The figure shows three views and two pictorial views of one solid part (mm, origin at its lowest corner). Answer the questions. Coordinates: 2 decimals unless noted, no trailing zeros. Loops run counter-clockwise (first coordinate to the right, second up) from the corner with the lowest first, then second, coordinate; pieces in that order, holes last.
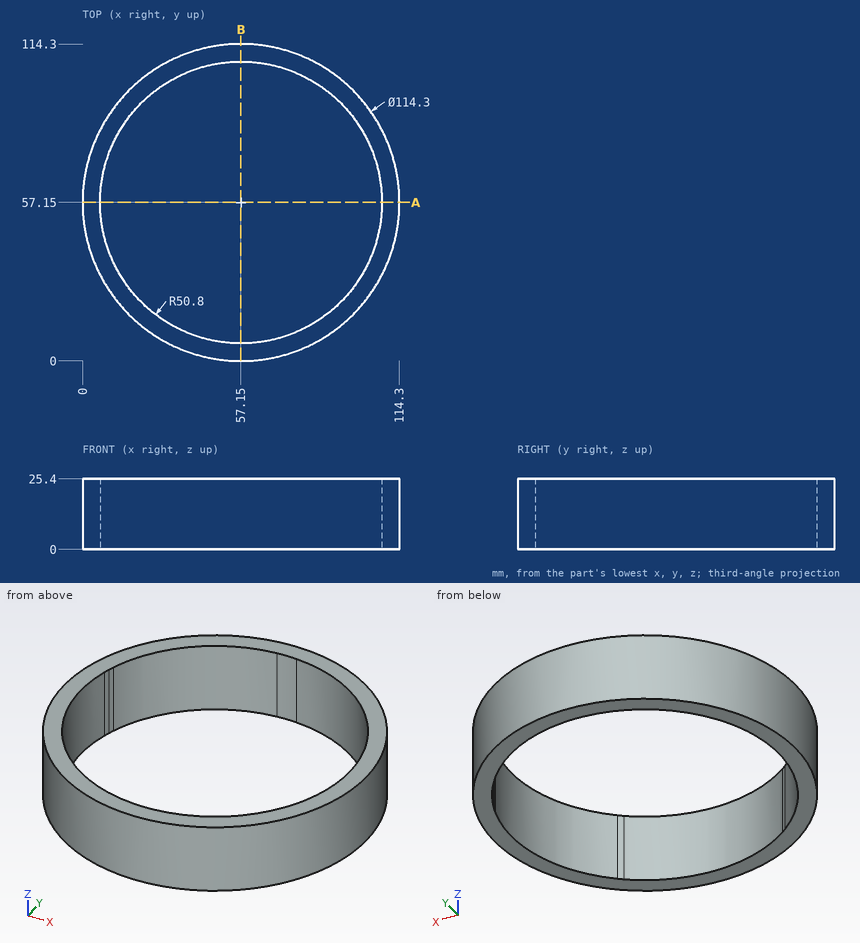
Q1. A cutting plane is placed at A-A (y = 57.15). Give the vertices of the cut face in (x, z).
Findings below:
outline: (0, 0) - (6.35, 0) - (6.35, 25.4) - (0, 25.4) - close; (107.95, 0) - (114.3, 0) - (114.3, 25.4) - (107.95, 25.4) - close
Q2. Flat-ended cylindrical pins translate along their axes: pin 1 Ø3 at (x, z) = (62, 8) entering from -Y; pin 2 Ø2 at (y, z) = (13.5, 20) entering from -X; pin 3 Ø1 at (x, z) = (26.5, 3) entering from +Y. Find the tip coordinate at first contact, or state that the pin passes through.
Findings below:
pin 1: stops at y = 0.1
pin 2: stops at x = 19.11
pin 3: stops at y = 105.7
Q3. Straight lines are drawn through the part: probe 1 along X at (y, z) = (30, 16); probe 2 along Y at (x, z) = (53, 7); probe 3 along X at (y, z) = (63.5, 22.75). For each, find the intervals that lie inside material, in ascending order.
Findings below:
probe 1: x = 6.86 to 14.21, 100.09 to 107.44
probe 2: y = 0.15 to 6.52, 107.78 to 114.15
probe 3: x = 0.35 to 6.75, 107.55 to 113.95
